from build123d import *

# Parameters (mm, degrees)
ESQUISSE1_R                  = 10.25
BOSS_EXTRU_1_DEPTH           = 1
D_GAGEMENT_M21_D             = 2.6
R_P_TITION_CIRCULAIRE1_COUNT = 4
ESQUISSE9_R                  = 5.5
BOSS_EXTRU_4_DEPTH           = 5
CONG_1_R                     = 0.5
ESQUISSE11_R                 = 4
ENL_V_MAT_EXTRU_2_DEPTH      = 5
BOSS_EXTRU_5_DEPTH           = 5


with BuildPart() as part:
    # Esquisse1 → Boss.-Extru.1 (new body)
    with BuildSketch(Plane.XZ.offset(38.601290575)):
        with Locations(Location((14.017249305, 17.25, 0), (0, 0, 270))):
            Circle(ESQUISSE1_R)
    extrude(amount=BOSS_EXTRU_1_DEPTH)

    # Dégagement M21 (through all)
    with Locations(Plane(origin=(0, -39.601290575, 0), x_dir=(-1, 0, 0), z_dir=(0, -1, 0))):
        with Locations((-11.415520349, -24.815117741)):
            d_gagement_m21 = Hole(D_GAGEMENT_M21_D / 2)

    # Répétition circulaire1: Dégagement M21 ×4 about axis
    r_p_tition_circulaire1_axis = Axis((14.017249305, 0, 17.25), (0, 1, 0))
    for i in range(1, R_P_TITION_CIRCULAIRE1_COUNT):
        add(d_gagement_m21.rotate(r_p_tition_circulaire1_axis, i * 360 / R_P_TITION_CIRCULAIRE1_COUNT), mode=Mode.SUBTRACT)

    # Esquisse9 → Boss.-Extru.4 (add)
    with BuildSketch(Plane(origin=(0, -39.601290575, 0), x_dir=(-1, 0, 0), z_dir=(0, -1, 0))):
        with Locations(Location((-14.017249305, -17.25, 0), (0, 0, 90))):
            Circle(ESQUISSE9_R)
    extrude(amount=BOSS_EXTRU_4_DEPTH)

    # Congé1
    cong_1_edges = [part.edges().sort_by_distance(p)[0] for p in [
        (14.017249305, -39.601290575, 22.75),
    ]]
    fillet(cong_1_edges, radius=CONG_1_R)

    # Esquisse11 → Enlèv. mat.-Extru.2 (cut)
    with BuildSketch(Plane(origin=(0, -38.601290575, 0), x_dir=(1, 0, 0), z_dir=(0, 1, 0))):
        with Locations(Location((14.017249305, -17.25, 0), (0, 0, 270))):
            Circle(ESQUISSE11_R)
    extrude(amount=-ENL_V_MAT_EXTRU_2_DEPTH, mode=Mode.SUBTRACT)

    # Esquisse10 → Boss.-Extru.5 (add)
    with BuildSketch(Plane.XZ.offset(44.601290575)):
        with BuildLine():
            Line((12.238907381, 19.85), (15.79559123, 19.85))
            ThreePointArc((15.79559123, 19.85), (14.017249305, 14.1), (12.238907381, 19.85))
        make_face()
    extrude(amount=BOSS_EXTRU_5_DEPTH)


solid = part.part
Could you check a few things on this model? Use its own coordinates, in mm. A direction names the side the tool comes from. Coordinates: 2 decimals unless noted, no trailing zeros. Order: outer loops, then holes, each group sorted by start corner. A loop starts at its lowest first (then second) coordinate and runs counter-clockwise, first axis right, second up.
Q1. Suppose I cut it at C-C on y = -45. Please give me the cut outline in (x, z).
Q2. Which directions (+Z, -Z, +X, -X, +Y, -Y) give clear straight access to the entire face, cutting with the end or side of a thin tool? Please do faces 1 (the cylindrical face through (15.669, -42.32, 12.004)), 2 (the flat face through (14, -43.601, 17)), 3 (the cylindrical face through (6.8, -39.1, 15.9)).
Q3. Thinking about a two-plate mould opening in X: for faces 4 (the cylindrical face through (10.091, -39.094, 7.782)), 5 (the cylindrical face through (16.72, -41.07, 14.3)), 6 (the flat face through (14, -47, 19.85)), which applies, released by +X, released by -X, zero draft, split by the parting line, or undercut?
Q4. Suppose I cut it at D-D on x = 23.25. Please give me the cut outline in (y, z), and give its area (3 significant figures).
Q5. Suppose I cut it at B-B on z = 10. Please give me the cut outline in (x, y).
Q6. Suppose I cut it at A-A on z = 17.25. Please give me the cut outline in (x, y).
Q7. Will these pins go through, and if not, where does the flat tip stop? pin 1 (3.5 mm diameter, centred on x = 6.45, z = 14.65, fed in from -Y); pin 2 (1.5 mm diameter, centred on y = -42.5, z = 17, fed in from -X); pin 3 (2 mm diameter, centred on x = 16.62, z = 9.68, fed in from +Y); pin 4 (1.5 mm diameter, centred on y = -45, z = 21, fed in from +X).
Q8. Please list where these lines run through material, in increasing order: L1, parallel to Z at x = 14, y = -41; L2, parallel to Y at x = 13.75, z = 23.25; L3, parallel to Y at x = 9.75, z = 15.5.
Answer:
1. outline: (12.24, 19.85) arc R3.15 ccw (long way) to (15.8, 19.85) - close
2. face 1: -Y
2. face 2: +Y
2. face 3: +Y, -Y
3. face 4: split by the parting line
3. face 5: undercut
3. face 6: zero draft
4. outline: (-39.6, 12.8) - (-38.6, 12.8) - (-38.6, 21.7) - (-39.6, 21.7) - close
4. area: 8.90 mm2
5. outline: (6.77, -39.6) - (15.36, -39.6) - (15.36, -38.6) - (6.77, -38.6) - close; (17.88, -39.6) - (21.26, -39.6) - (21.26, -38.6) - (17.88, -38.6) - close
6. outline: (3.77, -39.6) - (8.02, -39.6) arc R0.5 cw to (8.52, -40.1) - (8.52, -44.6) - (10.87, -44.6) - (10.87, -49.6) - (17.17, -49.6) - (17.17, -44.6) - (19.52, -44.6) - (19.52, -40.1) arc R0.5 cw to (20.02, -39.6) - (24.27, -39.6) - (24.27, -38.6) - (18.02, -38.6) - (18.02, -43.6) - (10.02, -43.6) - (10.02, -38.6) - (3.77, -38.6) - close
7. pin 1: stops at y = -39.6
7. pin 2: stops at x = 8.52
7. pin 3: passes through
7. pin 4: stops at x = 18.55
8. L1: z = 11.75 to 13.25, 21.25 to 22.75
8. L2: y = -39.6 to -38.6
8. L3: y = -44.6 to -38.6
